from build123d import *

# Parameters (mm, degrees)
EXTRUDE_THIN1_DEPTH = 134.9375


with BuildPart() as part:
    # Sketch1 → Extrude-Thin1 (new, symmetric)
    with BuildSketch(Plane(origin=(0, 0, 0), x_dir=(0, 0, -1), z_dir=(1, 0, 0))):
        with BuildLine():
            ThreePointArc((24.209375, 95.25), (136.32181049, -122.691603728), (378.820833581, -158.215745192))
            ThreePointArc((378.820833581, -158.215745192), (388.767577151, -155.705127985), (398.991457096, -154.860625))
            Line((398.991457096, -154.860625), (620.869080778, -154.860625))
            ThreePointArc((620.869080778, -154.860625), (629.002086236, -155.393690341), (636.995933716, -156.983765468))
            Line((636.995933716, -156.983765468), (661.530449704, -163.557769213))
            Line((661.530449704, -163.557769213), (662.146762555, -161.257658339))
            Line((662.146762555, -161.257658339), (637.612246567, -154.683654594))
            ThreePointArc((637.612246567, -154.683654594), (629.312901731, -153.032812265), (620.869080778, -152.479375))
            Line((620.869080778, -152.479375), (398.991457096, -152.479375))
            ThreePointArc((398.991457096, -152.479375), (388.376855625, -153.356151985), (378.049981727, -155.962716346))
            ThreePointArc((378.049981727, -155.962716346), (137.706505507, -120.754345029), (26.590625, 95.25))
            Line((26.590625, 95.25), (24.209375, 95.25))
        make_face()
    extrude(amount=EXTRUDE_THIN1_DEPTH, both=True)


solid = part.part
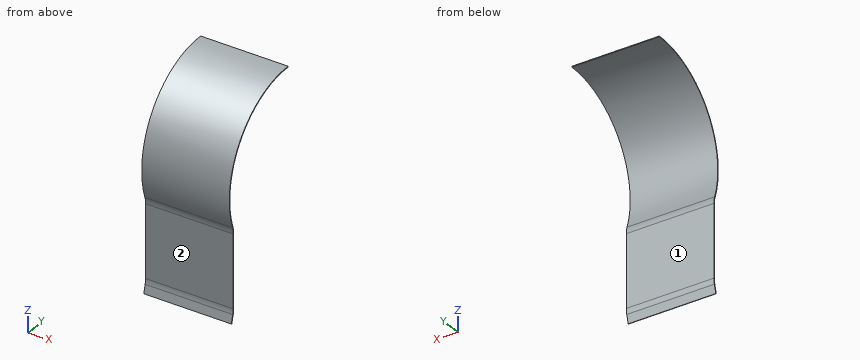
Model file for the job. Use its own axes, mm. Face numbers are marked on the shaded views. Coordinates: 2 decimals unless noted, no trailing zeros. Order: outer loops, then holes, each group sorted by start corner. A loop starts at its lowest first (then second) coordinate and runs counter-clockwise, first axis right, second up. Notation, with made-up numbers: (38, 35) -> (44, 35) arc R14 cw to (44, 62) -> close; hole circle Ø11 at (-4.5, -2). An arc over 180 degrees is marked (long way). Return JSON: item names as keys, results as strings. Group by question number.
Item 1: Wall check: line 1 along Y through (x, z) = (114.5, -422.5); line 2 along Y through (x, z) = (95.5, -277); line 3 along Z through (x, y) = (-91, 38). Give the ranges that are in metal, low to high. Write a range as [from, to].
Item 2: Flat gauge pins, fed straight in: P1, Ø2, axis at x = 10.5, z = -417.5, coming from the -Y side; P2, Ø2, axis at x = -48, y = 64, coming from the -Z side; P3, Ø1.5, axis at x = -17, y = -37, coming from the +Z side. Where does each tip first touch, or does it go through?
Item 3: Saw through at A-A on x = -91.5. Write the cut outline in (y, z).
Item 4: Saw through at C-C on y = -72.5. Write the cut outline in (x, z).
Item 5: Pull direction Z, two halves, no side cores. Call the marked faces 1 and 2: pulls with the +Z half, pulls with the -Z half, needs draft (parallel to the pull), parting line crosses it, or undercut.
Item 6: Saw through at B-B on z = -571.5. Write the cut outline in (x, y), then the cut area to 3 significant figures.
Values found:
{
 "1": {"line 1": "y = [-154.86, -152.48]", "line 2": "y = [-172.21, -169.83]", "line 3": "z = [-32.84, -30.4]"},
 "2": {"P1": "stops at y = -154.86", "P2": "stops at z = -28.56", "P3": "stops at z = -58.71"},
 "3": {"outline": "(-163.56, -661.53) -> (-161.26, -662.15) -> (-154.68, -637.61) arc R64.69 ccw to (-152.48, -620.87) -> (-152.48, -398.99) arc R64.69 ccw to (-155.96, -378.05) arc R265.51 cw to (95.25, -26.59) -> (95.25, -24.21) arc R267.89 ccw to (-158.22, -378.82) arc R62.31 cw to (-154.86, -398.99) -> (-154.86, -620.87) arc R62.31 cw to (-156.98, -637) -> close"},
 "4": {"outline": "(-134.94, -86.3) -> (134.94, -86.3) -> (134.94, -83.23) -> (-134.94, -83.23) -> close"},
 "5": {"face 1": "needs draft", "face 2": "undercut"},
 "6": {"outline": "(-134.94, -154.86) -> (134.94, -154.86) -> (134.94, -152.48) -> (-134.94, -152.48) -> close", "area": "643 mm2"}
}
